Answer from the drawing. Dimensions are ordinates in mm from the lowest x, y and z of the part. Round coordinates to 2 decimals unless told otherwise and drop trailing zeros. Write each loop counter-clockwise with the first axis right and the second up, starting at its lowest first coordinate (ties: lowest second). Pieces come first, ordered by that corner, then holes. Notation, with made-up numbers: (-5, -2) - (39, -2) arc R15 ccw to (39, 9) - close; hole circle Ø4 at (-21.5, 6). An arc over 180 degrees is marked (long way). Answer as CSV lines item,"result". Start each with the question number.
1) Each of these flat-tipped pins is pushed along its axis until it touches: pin 1 (2 mm diameter, centred on y = 109, z = 25, fed in from +X); pin 2 (6 mm diameter, centred on x = 512, z = 44, fed in from -Y); pin 3 (4 mm diameter, centred on x = 208, z = 138, fed in from -Y) (1 decimal). Where does it stop, or does it pass through?
2) Find section C-C on x = 164.5. Determine the outline of the cut face in (y, z).
3) Consider line 1 along Y through (x, z) = (603, 158.5); line 2 along X through (y, z) = (225.5, 43) (1 decimal); line 3 along X through (y, z) = (82.5, 162) (1 decimal). Determine where each line is inside the solid, lowest interval first.
4) Find section B-B on y = 136. Determine the outline of the cut face in (x, z) (1 decimal).
5) Find section A-A on z = 79. Determine the outline of the cut face in (x, y).
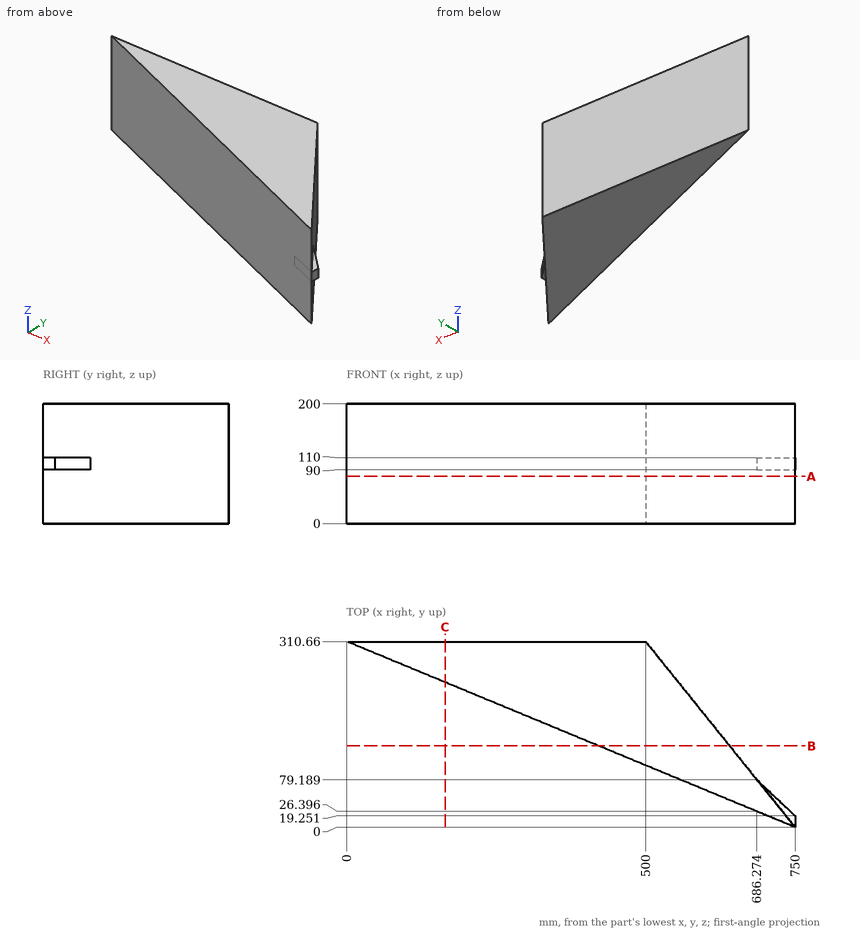
Check values:
1,pin 1,"stops at x = 663.09"
1,pin 2,"stops at y = 97.34"
1,pin 3,"stops at y = 223.7"
2,outline,"(242.52, 0) - (310.66, 0) - (310.66, 200) - (242.52, 200) - close"
3,line 1,"y = 60.89 to 182.67"
3,line 2,"x = 205.6 to 568.5"
3,line 3,"x = 550.8 to 683.6"
4,outline,"(421.7, 0) - (640.6, 0) - (640.6, 200) - (421.7, 200) - close"
5,outline,"(0, 310.66) - (750, 0) - (500, 310.66) - close"
